Work out the finished part from the listing and answer in its coordinate system (mm). A direction names the side the tool comes from. Round coordinates to 2 decimals unless told otherwise and drop trailing zeros. Loops run counter-clockwise (first coordinate to the right, second up) from the corner with the lowest first, then second, coordinate; pieces in that order, holes last. Notation, with made-up numbers: (56, 21.25) -> (107, 21.25) arc R25 cw to (107, 34.25) -> close; hole circle Ø9 at (70.5, 78.25). An arc over 180 degrees is marked (long way). Use one line per item in the form item = value.
Autodesk Fusion 360 part; units mm, degrees
sketch "Esquisse1" plane through (0, 0, 0) normal (0, 1, 0) x (1, 0, 0)
  circle A0 centre (0, 0) radius 45
  dimension "d1" = 90
sketch "Esquisse2" plane through (0, 0, 0) normal (0, 1, 0) x (1, 0, 0)
  circle A0 centre (0, 0) radius 43
  dimension "d2" = 86
sketch "Esquisse3" plane through (0, 0, 0) normal (0, 1, 0) x (1, 0, 0)
  circle A0 centre (0, 0) radius 35.5
  dimension "d3" = 71
extrude "Extrusion1" add sketch "Esquisse1" along normal blind 70 draft -26
sketch "Esquisse4" plane through (0, 70, 0) normal (0, 1, 0) x (-1, 0, 0)
  circle A0 centre (0, 0) radius 10.8587
  circle A1 centre (0, 0) radius 5
  dimension "d6" = 10
extrude "Extrusion2" cut sketch "Esquisse2" along normal blind 5 draft -26
extrude "Extrusion3" cut sketch "Esquisse4" against normal blind 15 contours A1
extrude "Extrusion4" cut sketch "Esquisse3" along normal blind 70 draft -26
sketch "Esquisse5" plane through (0, 0, 0) normal (0, 0, 1) x (1, 0, 0)
(1) Consider L1, parallel to Z at x = 0, y = 65; L2, parallel to Z at x = 0, y = 66; L3, parallel to X at y = 68, z = 0. Determine where each line is inside the solid, lowest interval first.
Completed:
L1 = -13.3 to -5, 5 to 13.3
L2 = -12.81 to -5, 5 to 12.81
L3 = -11.83 to -5, 5 to 11.83
(2) Find section D-D, the plane y = 40.5. Write down the section's boundary in (x, z).
Completed:
outline = circle Ø50.49 at (0, 0); hole circle Ø31.49 at (0, 0)
(3) Find section A-A, the plane x = 0. Write down the section's boundary in (y, z), then the cut area to 3 significant figures.
Completed:
outline = (0, -45) -> (70, -10.86) -> (70, -5) -> (62.53, -5) -> (5, -33.06) -> (5, -40.56) -> (0, -43) -> close; (0, 43) -> (5, 40.56) -> (5, 33.06) -> (62.53, 5) -> (70, 5) -> (70, 10.86) -> (0, 45) -> close
area = 1,230 mm2
(4) Find section B-B, the plane z = 0. Write down the section's boundary in (x, y).
Completed:
outline = (-45, 0) -> (-43, 0) -> (-40.56, 5) -> (-33.06, 5) -> (-5, 62.53) -> (-5, 70) -> (-10.86, 70) -> close; (5, 62.53) -> (33.06, 5) -> (40.56, 5) -> (43, 0) -> (45, 0) -> (10.86, 70) -> (5, 70) -> close
(5) Given P1, Ø6, axis at x = -17, z = -34, coming from the +Y side; P2, Ø12, axis at x = -22.5, z = 21, coming from the +Y side; P3, Ø5, axis at x = -21.5, z = 22, coming from the +Y side, each flat-ended and moving along its own axis, determine where each tip first touches the part or whether it passes through.
Completed:
P1 = 20.48
P2 = 41.46
P3 = 34.32
(6) Find section C-C, the plane y = 13.5. Write down the section's boundary in (x, z).
Completed:
outline = circle Ø76.83 at (0, 0); hole circle Ø57.83 at (0, 0)
(7) For faces 1 (the flat face through (23.1, 0, 36.5)), 2 (the flat face through (-33.24, 5, -0.19)), determine the directions among +Z, -Z, +X, -X, +Y, -Y from which every point of the face is accessible in a straight line to the end or side of a thin tool.
Completed:
face_1 = +Z, -Z, +X, -X, -Y
face_2 = -Y
